Verification items for the finished model (mm, model axes). A direction names the side the tool comes from. Give positions to 0.01 mm unless a question says otherwise; leave off trailing zeros. Write each loop counter-clockwise with the first axis right and the second up, starting at its lowest first coordinate (ties: lowest second). Pieces come first, ordered by that corner, then holes. Notation, with made-up numbers: (54, 62.5) - (64, 62.5) arc R35 ccw to (64, 96.5) - close; hole circle Ø9 at (-35.5, 61.5). An arc over 180 degrees is marked (long way). Put each result on its own line as item: value.
from build123d import *

# Parameters (mm, degrees)
F0_W      = 127.7551352978
F0_H      = 88.7857824564
F1_DEPTH  = 230
F4_DEPTH  = 20
F5_DEPTH  = 19.9898
F6_W      = 26.9565298222
F6_H      = 173.913128674
F6_W_2    = 6.0869585723
F6_H_2    = 140.0000751019
F7_DEPTH  = 4.826
F8_SIZE   = 5.08
F9_R      = 13.0796675924
F9_R_2    = 11.2186028003
F9_W      = 5.2173919976
F9_H      = 53.9130866528
F10_DEPTH = 4.826
F11_R     = 2.54


with BuildPart() as f1:
    # F0 (on Top) → F1 (new body)
    with BuildSketch(Plane.XY):
        Rectangle(F0_W, F0_H)
    extrude(amount=F1_DEPTH)

    # F3 (on face) → F4 (join)
    with BuildSketch(Plane.XZ.offset(44.3928912282)):
        Polygon((-41.2921301063, 173.0379974811), (-41.085819379, 172.688162985), (-41.1297441764, 172.6104329043), (-40.9572269026, 172.3179008855), (-18.8467815635, 172.5222300093), (-18.8301746286, 172.5516179285), (-19.2372092384, 173.2418134869), align=None)
        Polygon((-40.9572269026, 172.3179008855), (-41.1297441764, 172.6104329043), (-51.9640878366, 153.4377910705), (-40.9382216824, 134.7415827759), (-18.8833008145, 134.9453987817), (-8.0050323569, 154.1957706962), (-18.8301746286, 172.5516179285), (-18.8467815635, 172.5222300093), align=None)
        Polygon((-41.3476545775, 173.0374843632), (-41.2921301063, 173.0379974811), (-52.1454789867, 191.4416737569), (-52.1894037841, 191.3639436762), (-41.3642615124, 173.008096444), align=None)
        Polygon((-52.1454789867, 191.4416737569), (-41.2921301063, 173.0379974811), (-19.2372092384, 173.2418134869), (-18.8301746286, 172.5516179285), (-7.968513106, 191.7726019238), (-19.2006899874, 210.8186447145), (-41.3111353265, 210.6143155907), align=None)
        Polygon((-40.9382216824, 134.7415827759), (-51.9640878366, 153.4377910705), (-52.0196123078, 153.4372779525), (-40.9937461536, 134.7410696579), align=None)
        Polygon((-52.225923035, 153.7871124486), (-41.3642615124, 173.008096444), (-52.1894037841, 191.3639436762), (-52.1454789867, 191.4416737569), (-52.3179962605, 191.7342057757), (-74.4284415995, 191.5298766519), (-85.3067100571, 172.2795047374), (-74.0745331757, 153.2334619467), (-52.0196123078, 153.4372779525), align=None)
        Polygon((-40.9937461536, 134.7410696579), (-52.0196123078, 153.4372779525), (-74.0745331757, 153.2334619467), (-84.9528016333, 133.9830900322), (-73.7206247518, 114.9370472415), (-52.1037964015, 115.1368147056), (-52.2374327127, 115.3634175206), (-41.3591642551, 134.6137894351), (-40.8655472663, 134.6183510948), (-40.9382216824, 134.7415827759), align=None)
        Polygon((-19.248718916, 134.8181185589), (-40.8655472663, 134.6183510948), (-40.7319109552, 134.3917482798), (-51.6101794127, 115.1413763653), (-52.1037964015, 115.1368147056), (-51.9623043786, 114.8968912116), (-51.4474166697, 114.9016494402), (-40.4903681222, 96.3221329585), (-18.8948104921, 96.5217038537), (-8.0165420346, 115.7720757682), align=None)
        Polygon((-40.7319109552, 134.3917482798), (-40.8655472663, 134.6183510948), (-41.3591642551, 134.6137894351), (-52.2374327127, 115.3634175206), (-52.1037964015, 115.1368147056), (-51.6101794127, 115.1413763653), align=None)
        Polygon((-41.0052558312, 96.3173747299), (-51.9623043786, 114.8968912116), (-73.5578620087, 114.6973203164), (-84.4361304663, 95.4469484019), (-73.2039535849, 76.4009056112), (-51.0935082458, 76.605234735), (-51.0213053835, 76.7330061684), (-51.2069400891, 77.0477809963), (-40.4008744938, 96.1703814775), (-40.4903681222, 96.3221329585), align=None)
        Polygon((-51.4474166697, 114.9016494402), (-51.9623043786, 114.8968912116), (-41.0052558312, 96.3173747299), (-40.4903681222, 96.3221329585), align=None)
        Polygon((-40.3286716315, 96.2981529109), (-40.4008744938, 96.1703814775), (-40.2152397882, 95.8556066495), (-51.0213053835, 76.7330061684), (-39.9747632076, 58.0017382056), (-17.8643178685, 58.2060673294), (-6.986049411, 77.4564392439), (-18.2182262924, 96.5024820346), align=None)
        Polygon((-40.2152397882, 95.8556066495), (-40.4008744938, 96.1703814775), (-51.2069400891, 77.0477809963), (-51.0213053835, 76.7330061684), align=None)
    extrude(amount=F4_DEPTH)

    # F2 (on face) → F5 (join)
    with BuildSketch(Plane.XZ.offset(44.3928912282)):
        Polygon((-52.6453907674, 191.9314519259), (-41.7671223098, 211.1818238404), (-52.9992991913, 230.2278666311), (-75.1097445304, 230.0235375074), (-85.9880129879, 210.7731655929), (-74.7558361065, 191.7271228021), align=None)
    extrude(amount=F5_DEPTH)

    # F6 (on face) → F7 (cut)
    with BuildSketch(Plane.YZ.offset(63.8775676489)):
        with Locations((-2.6086920407, 121.6356754303)):
            Rectangle(F6_W, F6_H)
        with Locations((-2.6086920407, 121.6356754303)):
            Rectangle(F6_W_2, F6_H_2, mode=Mode.SUBTRACT)
    extrude(amount=-F7_DEPTH, mode=Mode.SUBTRACT)

    # F8
    f8_edges = [f1.edges().sort_by_distance(p)[0] for p in [
        (5.506325, -44.392891, 230),
        (63.877568, 0, 230),
        (0, 44.392891, 230),
        (-63.877568, 0, 230),
    ]]
    chamfer(f8_edges, length=F8_SIZE)

    # F9 (on face) → F10 (join)
    with BuildSketch(Plane.XZ.offset(44.3928912282)):
        with Locations((30.683927238, 69.0269544721)):
            Circle(F9_R)
        with Locations((28.9447959512, 108.1574112177)):
            Circle(F9_R_2)
        with Locations((11.5534868091, 164.2443984747)):
            Rectangle(F9_W, F9_H)
        Polygon((27.5010903101, 149.4617760181), (42.562418737, 149.4617760181), (50.0930829504, 162.5052690506), (42.562418737, 175.5487620831), (27.5010903101, 175.5487620831), (19.9704260966, 162.5052690506), align=None)
    extrude(amount=F10_DEPTH)

    # F11
    f11_edges = [f1.edges().sort_by_distance(p)[0] for p in [
        (35.031755, -49.218891, 175.548762),
        (46.327751, -49.218891, 155.983523),
        (35.031755, -49.218891, 149.461776),
        (23.735758, -49.218891, 155.983523),
        (23.735758, -49.218891, 169.027016),
        (17.726193, -49.218891, 108.157411),
        (17.60426, -49.218891, 69.026954),
    ]]
    fillet(f11_edges, radius=F11_R)


solid = f1.part
Q1. Section check A-A, the plane y = -54. Give the number of separate pieces and of enclosed holes in the cut face, plus the area to 3 significant figures.
Answers follow:
separate pieces: 2
enclosed holes: 1
area: 10,100 mm2
Q2. Set-up check for faces 1 (the face through (12, -49.219, 165)), 2 (the face through (61, -3, 208.592)), 3 (the face through (-47.282, -54.248, 201.422)), 4 (the face through (12, -47, 137.288)): record each of +Z, -Z, +X, -X, +Y, -Y from which the full face is reachable in a straight line by a thin tool's end or side.
Answers follow:
face 1: +Z, -Z, +X, -Y
face 2: +X
face 3: -Y
face 4: -Z, +X, -Y
Q3. Section check C-C, the plane y = 5. Record the cut outline in (x, z).
Answers follow:
outline: (-63.88, 0) - (63.88, 0) - (63.88, 34.68) - (59.05, 34.68) - (59.05, 208.59) - (63.88, 208.59) - (63.88, 224.92) - (58.8, 230) - (-58.8, 230) - (-63.88, 224.92) - close
Q4. Release check for a two-part mould opening along X. For faces 5 (the face through (61, -3, 191.636)), 6 (the face through (-63.878, -1, 111)), 7 (the face through (-12.5, -54.3, 67.7)) record: released by +X, released by -X, zero draft, split by the parting line, or undercut.
Answers follow:
face 5: zero draft
face 6: released by -X
face 7: undercut
Q5. Scan lines: line 1 along Y through (x, z) = (-13.5, 48); line 2 along X through (y, z) = (-40, 208); line 3 along Z through (x, y) = (16, -4). Record each from-to range of solid material in increasing order.
Answers follow:
line 1: y = -44.39 to 44.39
line 2: x = -63.88 to 63.88
line 3: z = 0 to 230
Q6. Section check B-B, the plane x = -70. Record the cut outline in (y, z).
Answers follow:
outline: (-64.39, 76.43) - (-44.39, 76.43) - (-44.39, 114.73) - (-64.39, 114.73) - close; (-64.39, 114.97) - (-44.39, 114.97) - (-44.39, 191.57) - (-64.39, 191.57) - close; (-64.38, 191.77) - (-44.39, 191.77) - (-44.39, 230.07) - (-64.38, 230.07) - close
Q7. Go/stop test with flat-tipped pins: pin 1 Ø2 at (x, y) = (-23, -4) entering from +Z; pin 2 Ø10 at (y, z) = (14.5, 132.5) entering from -X; pin 3 Ø1.5 at (x, z) = (-15.5, 29.5) entering from -Y; pin 4 Ø5.5 at (x, y) = (62.5, -3) entering from -Z. Record where each tip stops, or that it passes through.
Answers follow:
pin 1: stops at z = 230
pin 2: stops at x = -63.88
pin 3: stops at y = -44.39
pin 4: stops at z = 0
Q8. Section check D-D, the plane z = 144.5. Record the cut outline in (x, y).
Answers follow:
outline: (-79.01, -64.39) - (-13.48, -64.39) - (-13.48, -44.39) - (8.94, -44.39) - (8.94, -49.22) - (14.16, -49.22) - (14.16, -44.39) - (63.88, -44.39) - (63.88, -16.09) - (59.05, -16.09) - (59.05, -5.65) - (63.88, -5.65) - (63.88, 0.43) - (59.05, 0.43) - (59.05, 10.87) - (63.88, 10.87) - (63.88, 44.39) - (-63.88, 44.39) - (-63.88, -44.39) - (-79.01, -44.39) - close
